Autodesk Inventor part; units mm, degrees
ref_plane "YZ Plane" through (0, 0, 0) normal (1, 0, 0) x (0, 1, 0)
ref_plane "XZ Plane" through (0, 0, 0) normal (0, 1, 0) x (-1, 0, 0)
ref_plane "XY Plane" through (0, 0, 0) normal (0, 0, 1) x (1, 0, 0)
sketch "Sketch1" plane through (0, 0, 0) normal (0, 0, 1) x (1, 0, 0)
  circle A0 centre (0, 0) radius 3.175
  dimension "d0" = 6.35
extrude "Extrusion1" add sketch "Sketch1" along normal blind 12.7
sketch "Sketch2" plane through (0, 0, 0) normal (0, 0, -1) x (-1, 0, 0)
  circle A0 centre (0, 0) radius 3.175
  circle A1 centre (0, 0) radius 4.7625
  dimension "d3" = 9.525
extrude "Extrusion2" add sketch "Sketch2" along normal blind 6.35 contours A0 | A1
sketch "Sketch3" plane through (0, 0, -6.35) normal (0, 0, -1) x (-1, 0, 0)
  circle A0 centre (0, 0) radius 4.7625
  line L0 (-1.3748, 2.3812) -> (1.3748, 2.3813)
  line L1 (1.3748, 2.3813) -> (2.7496, 0)
  line L2 (2.7496, 0) -> (1.3748, -2.3812)
  line L3 (1.3748, -2.3812) -> (-1.3748, -2.3812)
  line L4 (-1.3748, -2.3812) -> (-2.7496, 0)
  line L5 (-2.7496, 0) -> (-1.3748, 2.3812)
  dimension "d6" = 4.7625
extrude "Extrusion3" cut sketch "Sketch3" against normal blind 3.175 contours L0 L1 L2 L3 L4 L5
chamfer "Chamfer1" distance 0.508 angle 45 3 edges at (-3.175, 0, 12.7) (4.7625, 0, 0) (4.7625, 0, -6.35)
thread "Thread1"
properties part number "14-20 x750" material "Steel"
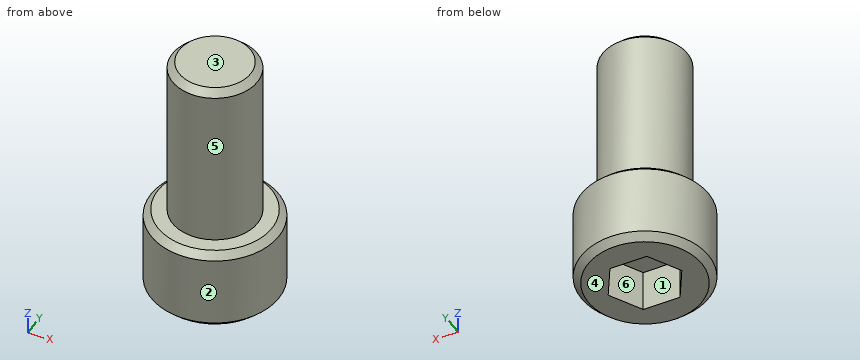
The listing builds one solid part. Answer for the finished solid, in the listing's coordinates (mm). Face numbers are marked on the shaded views. A direction names the side the tool comes from. Give positions to 0.01 mm unless a question says otherwise; leave off trailing zeros. Loops run counter-clockwise (first coordinate to the right, second up) from the corner with the lowest first, then second, coordinate; pieces in that order, holes last. Notation, with made-up numbers: (33, 47.25) - (76, 47.25) arc R16 cw to (76, 57.25) - close; hole circle Ø7 at (-39.75, -17). An arc over 180 degrees is marked (long way). Return JSON: item names as keys, results as strings. Group by question number.
1. Straight lines are drawn through the part: line 1 (Z direction, x = 4, y = -0.75); line 2 (Z direction, x = -2.5, y = 0.25) (3 decimals); line 3 (Y direction, x = 0, z = 11.75) (3 decimals). For each, find the intervals that lie inside material, in ascending order. Write a range as [from, to].
2. Find section B-B (z = -1.5). Write down the section's boundary in (x, y) (1 decimal).
3. Find section C-C (z = 10.75). Write down the section's boundary in (x, y) (3 decimals).
4. Given pin 1 Ø2 at (x, z) = (3.5, -4) entering from +Y; pin 2 Ø4 at (y, z) = (-2, 5) entering from +X (3 decimals); pin 3 Ø1.5 at (y, z) = (0, 1) entering from -X (3 decimals), each flat-ended and moving along its own axis, determine where each tip first touches the part or whether it passes through.
5. Which of the six approach directions +Z, -Z, +X, -X, +Y, -Y give full straight-line access (tool end or side, diameter ignored) to the marked faces 4, 5 and 6?
6. Determine the mould class of the marked faces 1, 2 and 3 for opening direction X: pulls with the +X half, pulls with the -X half, needs draft (parallel to the pull), parting line crosses it, or undercut.
Verdict:
{
 "1": {"line 1": "z = [-6.35, 0]", "line 2": "z = [-3.175, 12.7]", "line 3": "y = [-3.175, 3.175]"},
 "2": {"outline": "circle Ø9.5 at (0, 0)"},
 "3": {"outline": "circle Ø6.35 at (0, 0)"},
 "4": {"pin 1": "stops at y = 4.05", "pin 2": "stops at x = 3.175", "pin 3": "stops at x = -3.175"},
 "5": {"face 4": "-Z, +X, -X, +Y, -Y", "face 5": "+Z", "face 6": "-Z"},
 "6": {"face 1": "undercut", "face 2": "parting line crosses it", "face 3": "needs draft"}
}
